The listing builds one solid part. Answer for the finished solid, in the listing's coordinates (mm). Give positions to 0.01 mm unless a question says otherwise; leave off trailing zeros. Write each loop counter-clockwise with the first axis right and the second up, starting at its lowest first coordinate (ties: lowest second). Pieces come first, ordered by that corner, then holes. Notation, with made-up numbers: (43.25, 74.25) -> (101.25, 74.25) arc R6 cw to (101.25, 80.25) -> close; hole circle Ø4 at (-22.75, 2.25). An arc over 180 degrees is marked (long way). Put each result on its own line as item: value. Start each with the question number.
1) A cutting plane is placed at C-C (x = 27). Write down the section's boundary in (y, z).
2) A cutting plane is placed at D-D (z = 87.5). Write down the section's boundary in (x, y), then the cut area to 4 significant figures.
3) A cutting plane is placed at B-B (z = 75). Write down the section's boundary in (x, y).
4) Find the intervals of material crossed by line 1 along X through (y, z) = (-4, 83); line 2 along Z through (x, y) = (20, -3.25); line 3 along Z through (x, y) = (55, -1), in increasing order. Write a range as from..to.
5) A flat-ended cylindrical pin translates along its axis: pin 1 Ø1 at (y, z) = (-1.5, 24.5) entering from -X. Find the tip coordinate at first contact, or state that the pin passes through.
6) A cutting plane is placed at A-A (y = -4.25). Write down the section's boundary in (x, z), then the cut area to 3 significant figures.
from build123d import *

# Parameters (mm, degrees)
F0_R        = 10
F1_DEPTH    = 10
F2_T1_DEPTH = 217
F2_T3_DEPTH = 230
F4_D        = 10.5


# Not quite as in the source:
# - a fillet or chamfer that OpenCascade refuses, or shapes differently, is made with other operations: its cross-section is extruded or revolved along the edge and cut away or added


with BuildPart() as f1:
    # F0 (on Front) → F1 (new body)
    with BuildSketch(Plane.XZ):
        with BuildLine():
            Line((0, 90), (0, 0))
            Line((0, 0), (220, 0))
            Line((220, 0), (220, 90))
            ThreePointArc((220, 90), (217.0710678119, 97.0710678119), (210, 100))
            Line((210, 100), (10, 100))
            ThreePointArc((10, 100), (2.9289321881, 97.0710678119), (0, 90))
        make_face()
        with Locations((20, 75)):
            Circle(F0_R, mode=Mode.SUBTRACT)
    extrude(amount=F1_DEPTH)

    # F2: fillet of radius 2 on 4 edges, made by hand

    # F2_s2 → F2_t1 (cut)
    with BuildSketch(Plane.YZ.offset(1.5)):
        with BuildLine():
            ThreePointArc((-8, 100), (-9.4142135624, 99.4142135624), (-10, 98))
            Line((-10, 98), (-10, 100))
            Line((-10, 100), (-8, 100))
        make_face()
        with BuildLine():
            ThreePointArc((-2, 100), (-0.5857864376, 99.4142135624), (0, 98))
            Line((0, 98), (0, 100))
            Line((0, 100), (-2, 100))
        make_face()
    extrude(amount=F2_T1_DEPTH, mode=Mode.SUBTRACT)

    # F2_s4 → F2_t3 (cut)
    with BuildSketch(Plane.YZ.offset(-5)):
        with BuildLine():
            ThreePointArc((-8, 0), (-9.4142135624, 0.5857864376), (-10, 2))
            Line((-10, 2), (-10, 0))
            Line((-10, 0), (-8, 0))
        make_face()
        with BuildLine():
            ThreePointArc((-2, 0), (-0.5857864376, 0.5857864376), (0, 2))
            Line((0, 2), (0, 0))
            Line((0, 0), (-2, 0))
        make_face()
    extrude(amount=F2_T3_DEPTH, mode=Mode.SUBTRACT)

    # F4 (through all)
    with Locations(Plane.XZ.offset(10)):
        with Locations((171.1133077741, 87.5)):
            Hole(F4_D / 2)


solid = f1.part
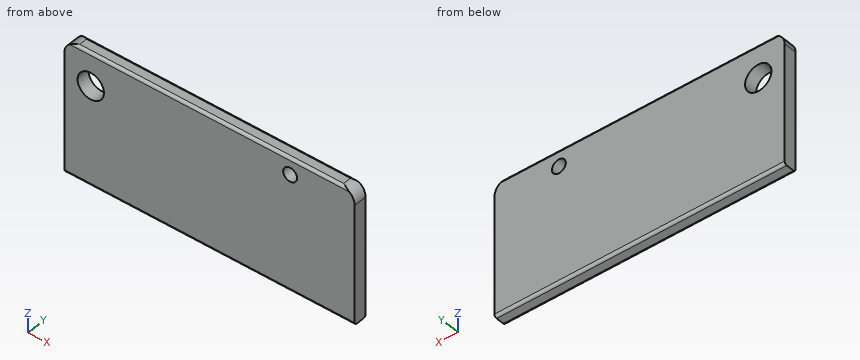
Reply:
1. outline: (-10, 2) arc R2 ccw to (-8, 0) -> (-2, 0) arc R2 ccw to (0, 2) -> (0, 67.86) -> (-10, 67.86) -> close; (-10, 82.14) -> (0, 82.14) -> (0, 98) arc R2 ccw to (-2, 100) -> (-8, 100) arc R2 ccw to (-10, 98) -> close
2. outline: (0, -10) -> (165.86, -10) -> (165.86, 0) -> (0, 0) -> close; (176.36, -10) -> (220, -10) -> (220, 0) -> (176.36, 0) -> close
2. area: 2,095 mm2
3. outline: (0, -10) -> (10, -10) -> (10, 0) -> (0, 0) -> close; (30, -10) -> (220, -10) -> (220, 0) -> (30, 0) -> close
4. line 1: x = 0..14, 26..168.41, 173.82..220
4. line 2: z = 0..65, 85..100
4. line 3: z = 0.27..99.73
5. pin 1: stops at x = 0
6. outline: (0, 0) -> (220, 0) -> (220, 90) arc R10 ccw to (210, 100) -> (10, 100) arc R10 ccw to (0, 90) -> close; hole circle Ø20 at (20, 75); hole circle Ø10.5 at (171.11, 87.5)
6. area: 21,600 mm2
